from build123d import *

# Parameters (mm, degrees)
BOSS_EXTRU_1_DEPTH         = 3
ESQUISSE2_R                = 1.5
BOSS_EXTRU_2_DEPTH         = 10
R_P_TITION_LIN_AIRE1_COUNT = 2
R_P_TITION_LIN_AIRE1_PITCH = 20
ESQUISSE3_R                = 1.5
ENL_V_MAT_EXTRU_1_DEPTH    = 10


with BuildPart() as part:
    # Esquisse1 → Boss.-Extru.1 (new body)
    with BuildSketch(Plane.XY):
        with BuildLine():
            Line((-15, 10), (15, 10))
            ThreePointArc((15, 10), (18.535533906, 8.535533906), (20, 5))
            Line((20, 5), (20, -10))
            Line((20, -10), (-20, -10))
            Line((-20, -10), (-20, 5))
            ThreePointArc((-20, 5), (-18.535533906, 8.535533906), (-15, 10))
        make_face()
    extrude(amount=BOSS_EXTRU_1_DEPTH)

    # Esquisse2 → Boss.-Extru.2 (add)
    with BuildSketch(Plane(origin=(20, 0, 0), x_dir=(0, 0, -1), z_dir=(1, 0, 0))):
        with BuildLine():
            Line((-3, -10), (-3.705882353, -11.323529412))
            ThreePointArc((-3.705882353, -11.323529412), (-1.5, -15), (0.705882353, -11.323529412))
            Line((0.705882353, -11.323529412), (0, -10))
            Line((0, -10), (-3, -10))
        make_face()
        with Locations(Location((-1.5, -12.5, 0), (0, 0, 90))):
            Circle(ESQUISSE2_R, mode=Mode.SUBTRACT)
    boss_extru_2 = extrude(amount=-BOSS_EXTRU_2_DEPTH)

    # Répétition linéaire1: Boss.-Extru.2 ×2
    with Locations(*[(-i * R_P_TITION_LIN_AIRE1_PITCH, 0, 0) for i in range(1, R_P_TITION_LIN_AIRE1_COUNT)]):
        add(boss_extru_2)

    # Esquisse3 → Enlèv. mat.-Extru.1 (cut)
    with BuildSketch(Plane.XY.offset(3)):
        with Locations((0, -4)):
            Circle(ESQUISSE3_R)
        with Locations((-14, 2)):
            Circle(ESQUISSE3_R)
        with Locations((14, 2)):
            Circle(ESQUISSE3_R)
    extrude(amount=-ENL_V_MAT_EXTRU_1_DEPTH, mode=Mode.SUBTRACT)


solid = part.part
The model under review builds one solid part; all positions refer to its coordinate system, in mm. A direction names the side the tool comes from. Round coordinates to 2 decimals unless told otherwise and drop trailing zeros. Write each loop counter-clockwise with the first axis right and the second up, starting at its lowest first coordinate (ties: lowest second). Pieces come first, ordered by that corner, then holes. Notation, with made-up numbers: M -24.75,-20.75 L -5.75,-20.75 A19 cw -5.75,-12.75 Z; hole C 26,76.5 d11. An arc over 180 degrees is marked long. Answer as CSV lines item,"result". Start each with the question number.
Q1. The part is to be moulded in two halves that separate along Y. For faces 4 (the face through (-10, -14, 0)), 5 (the face through (-19, 8, 1)), 6 (the face through (-4.93, -14, 1.57)), 7 (the face through (-15.5, 2.07, 1.52)), say which applies: +Y half, -Y half, draft (parallel to the pull), parting line (faces both ways), or undercut.
Q2. Clearance check with flat-ended pins moving along their axes: P1, Ø2.5, axis at x = 0, y = -4, coming from the -Z side; P2, Ø0.9, axis at x = -13, z = 1, coming from the -Y side; P3, Ø3, axis at x = 14, y = -7, coming from the +Z side; P4, Ø6, axis at x = 5, y = -5, coming from the -Z side. State where each tip first meets the part, or that it passes through.
Q3. Wall thickness on line 1 along X through (y, z) = (-11.5, 3.1); line 2 along Z through (x, y) = (12.5, -8); line 3 along Y through (x, z) = (-11, 2.1): over which ranges is each line inside the solid? List them lowest first.
Q4. Consider section A-A, the plane z = 1.5. Give the boundary of the cut face in (x, y), then the cut area to 3 significant figures.
Q5. Consider section C-C, the plane x = -14. Give the boundary of the cut face in (y, z).
Q6. Consider section B-B, the plane y = -4. Give the boundary of the cut face in (x, z).
Q7. Tool access review of faces 1 (the face through (-15, -10, 1)), 2 (the face through (0, 0, 3)), 3 (the face through (0, 0, 0)): name each direction out of +Z, -Z, +X, -X, +Y, -Y from which nothing blocks a thin tool from reaching the whole face with its end or side.
Q8. Consider section D-D, the plane y = 2. Give the boundary of the cut face in (x, z).
Result set:
1,face 4,"draft"
1,face 5,"+Y half"
1,face 6,"undercut"
1,face 7,"undercut"
2,P1,"passes through"
2,P2,"stops at y = -10"
2,P3,"stops at z = 3"
2,P4,"stops at z = 0"
3,line 1,"x = -10 to 0, 10 to 20"
3,line 2,"z = 0 to 3"
3,line 3,"y = -10 to 10"
4,outline,"M -20,-10 L -10,-10 L -10,-11 L 0,-11 L 0,-10 L 10,-10 L 10,-11 L 20,-11 L 20,5 A5 ccw 15,10 L -15,10 A5 ccw -20,5 Z; M -10,-15 L 0,-15 L 0,-14 L -10,-14 Z; M 10,-15 L 20,-15 L 20,-14 L 10,-14 Z; hole C -14,2 d3; hole C 0,-4 d3; hole C 14,2 d3"
4,area,"808 mm²"
5,outline,"M -10,0 L 0.5,0 L 0.5,3 L -10,3 Z; M 3.5,0 L 10,0 L 10,3 L 3.5,3 Z"
6,outline,"M -20,0 L -1.5,0 L -1.5,3 L -20,3 Z; M 1.5,0 L 20,0 L 20,3 L 1.5,3 Z"
7,face 1,"+Z, -Z, -X, -Y"
7,face 2,"+Z, +X, -X, +Y"
7,face 3,"-Z, +X, -X, +Y"
8,outline,"M -20,0 L -15.5,0 L -15.5,3 L -20,3 Z; M -12.5,0 L 12.5,0 L 12.5,3 L -12.5,3 Z; M 15.5,0 L 20,0 L 20,3 L 15.5,3 Z"
